Can you work these out from the model? Positions are in its coordinate system, mm. A direction names the side the tool comes from. Round coordinates to 2 decimals unless told otherwise and drop trailing zeros. Write each loop counter-clockwise with the first axis right and the second up, starting at its lowest first coordinate (ties: lowest second). Pieces come first, ordered by that corner, then holes.
Q1. If we section it at D-D (x = -13): Please give me the cut outline in (y, z), plus the area to 3 significant figures.
Q2. If we section it at C-C (y = -22.25): Please give me the cut outline in (x, z).
Q3. I'm going to push flat-ended pins straight in: pin 1 Ø2.5 at (y, z) = (-21.5, 3) entering from +X; pin 2 Ø4.5 at (y, z) = (-30, 17) entering from +X; pin 3 Ø5.5 at (x, y) = (-18.5, -21) entering from +Z. Where does each tip first touch, or does it pass through?
Q4. For faces 1 (the flat face through (-22.804, -20, 2)), 2 (the flat face through (-4, -11, 6.65)), 3 (the cylindrical face through (-44.948, -30.565, 22.098)), which set-ups out of +Z, -Z, +X, -X, +Y, -Y let a thin tool reach every point of the face, with its end or its side?
Q5. Please list where these lines run through material, in increasing order: line 1 along Z through (x, y) = (-21, -16.75); line 2 along X through (y, z) = (-31.25, 10.25); line 3 along Y through (x, z) = (-7.5, 8.25).
Q6. If we section it at B-B (x = -32): Please give me the cut outline in (y, z).
Q7. If we section it at A-A (z = 11.5): Please give me the cut outline in (x, y), plus the area to 3 significant figures.
from build123d import *

# Parameters (mm, degrees)
F1_DEPTH  = 5
F0_W      = 23
F0_H      = 4
F2_DEPTH  = 23
F4_R      = 3
F3_R      = 9.5
F5_DEPTH  = 25
F0_W_2    = 15
F6_DEPTH  = 10
F7_R      = 2
F9_DEPTH  = 25
F10_DEPTH = 25
F11_R     = 1.5


with BuildPart() as f1:
    # F0 (on Top) → F1 (new body)
    with BuildSketch(Plane.XY):
        Polygon((-15.8038523793, -12.5927883387), (-15.8038523793, -8.5927883387), (-22.8038523793, -8.5927883387), (-22.8038523793, -28.5927883387), (-22.8038523793, -32.5927883387), (-15.8038523793, -32.5927883387), align=None)
    extrude(amount=F1_DEPTH)

    # F0 (on Top) → F2 (join)
    with BuildSketch(Plane.XY):
        with Locations((-34.3038523793, -30.5927883387)):
            Rectangle(F0_W, F0_H)
    extrude(amount=F2_DEPTH)

    # F4
    f4_edges = [f1.edges().sort_by_distance(p)[0] for p in [
        (-22.803852, -30.592788, 5),
        (-22.803852, -30.592788, 23),
        (-45.803852, -30.592788, 23),
        (-45.803852, -30.592788, 0),
        (-22.803852, -8.592788, 2.5),
        (-15.803852, -32.592788, 2.5),
    ]]
    fillet(f4_edges, radius=F4_R)

    # F3 (on face) → F5 (cut)
    with BuildSketch(Plane.XZ.offset(32.5927883387)):
        with Locations((-34.3038523793, 11.5)):
            Circle(F3_R)
    extrude(amount=-F5_DEPTH, mode=Mode.SUBTRACT)

    # F0 (on Top) → F6 (join)
    with BuildSketch(Plane.XY):
        with Locations((-8.3038523793, -10.5927883387)):
            Rectangle(F0_W_2, F0_H)
    extrude(amount=F6_DEPTH)

    # F7
    f7_edges = [f1.edges().sort_by_distance(p)[0] for p in [
        (-15.803852, -10.592788, 5),
        (-15.803852, -10.592788, 10),
        (-0.803852, -10.592788, 10),
        (-0.803852, -10.592788, 0),
    ]]
    fillet(f7_edges, radius=F7_R)

    # F8 (on face) → F9 (cut)
    with BuildSketch(Plane(origin=(0, -8.5927883387, 0), x_dir=(-1, 0, 0), z_dir=(0, 1, 0))):
        with BuildLine():
            ThreePointArc((5.7965948978, 3.350015961), (6.9680098333, 3.8307107192), (7.4538523793, 5))
            ThreePointArc((7.4538523793, 5), (6.9705785683, 6.166726189), (5.8038523793, 6.65))
            ThreePointArc((5.8038523793, 6.65), (4.1538563696, 5.0036287496), (5.7965948978, 3.350015961))
        make_face()
    extrude(amount=-F9_DEPTH, mode=Mode.SUBTRACT)

    # F8 (on face) → F10 (cut)
    with BuildSketch(Plane(origin=(0, -8.5927883387, 0), x_dir=(-1, 0, 0), z_dir=(0, 1, 0))):
        with BuildLine():
            ThreePointArc((5.7965948978, 3.350015961), (4.1538563696, 5.0036287496), (5.8038523793, 6.65))
            Line((5.8038523793, 6.65), (0.8038523793, 6.65))
            Line((0.8038523793, 6.65), (0.8038523793, 3.350015961))
            Line((0.8038523793, 3.350015961), (5.7965948978, 3.350015961))
        make_face()
    extrude(amount=-F10_DEPTH, mode=Mode.SUBTRACT)

    # F11
    f11_edges = [f1.edges().sort_by_distance(p)[0] for p in [
        (-0.803852, -10.592788, 3.350016),
        (-0.803852, -10.592788, 6.65),
    ]]
    fillet(f11_edges, radius=F11_R)


solid = f1.part
A:
1. outline: (-12.59, 0) - (-8.59, 0) - (-8.59, 10) - (-12.59, 10) - close
1. area: 40.0 mm2
2. outline: (-22.8, 0) - (-15.8, 0) - (-15.8, 5) - (-22.8, 5) - close
3. pin 1: stops at x = -15.8
3. pin 2: stops at x = -22.8
3. pin 3: stops at z = 5
4. face 1: +Z, -Z, -X, +Y
4. face 2: +X, +Y, -Y
4. face 3: +Z, -X, +Y, -Y
5. line 1: z = 0 to 5
5. line 2: x = -45.8 to -43.72, -24.89 to -22.8
5. line 3: y = -12.59 to -8.59
6. outline: (-32.59, 0) - (-28.59, 0) - (-28.59, 2.28) - (-32.59, 2.28) - close; (-32.59, 20.72) - (-28.59, 20.72) - (-28.59, 23) - (-32.59, 23) - close
7. outline: (-45.8, -32.59) - (-43.8, -32.59) - (-43.8, -28.59) - (-45.8, -28.59) - close; (-24.8, -32.59) - (-22.8, -32.59) - (-22.8, -28.59) - (-24.8, -28.59) - close
7. area: 16.0 mm2
